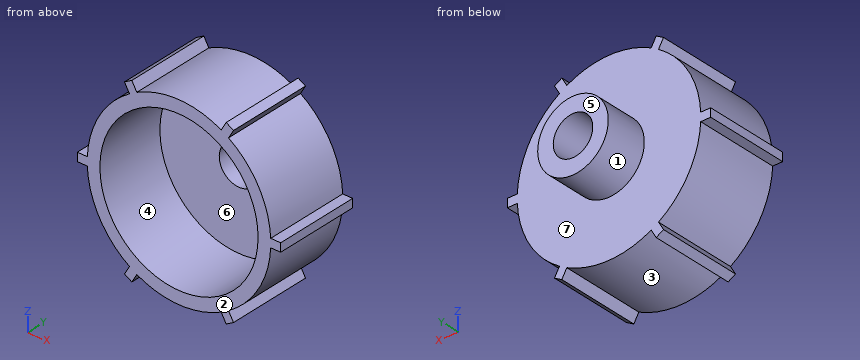
Autodesk Inventor part; units mm, degrees
ref_plane "YZ Plane" through (0, 0, 0) normal (1, 0, 0) x (0, 1, 0)
ref_plane "XZ Plane" through (0, 0, 0) normal (0, 1, 0) x (-1, 0, 0)
ref_plane "XY Plane" through (0, 0, 0) normal (0, 0, 1) x (1, 0, 0)
sketch "スケッチ1" plane through (0, 0, 0) normal (0, 1, 0) x (-1, 0, 0)
  circle A0 centre (0, 0) radius 6.5
  line L0 (0, 0) -> (0, -6.5) construction
  line L1 (3.5063, -5.4732) -> (2.9867, -5.7732)
  line L2 (2.9867, -5.7732) -> (3.3402, -6.3854)
  line L3 (3.3402, -6.3854) -> (3.8598, -6.0854)
  line L4 (3.8598, -6.0854) -> (3.5063, -5.4732)
  line L5 (0, 0) -> (3.6, -6.2354) construction
  line L6 (6.4931, 0.3) -> (6.4931, -0.3)
  line L7 (6.4931, -0.3) -> (7.2, -0.3)
  line L8 (7.2, -0.3) -> (7.2, 0.3)
  line L9 (7.2, 0.3) -> (6.4931, 0.3)
  line L10 (0, 0) -> (7.2, 0) construction
  line L11 (2.9867, 5.7732) -> (3.5063, 5.4732)
  line L12 (3.5063, 5.4732) -> (3.8598, 6.0854)
  line L13 (3.8598, 6.0854) -> (3.3402, 6.3854)
  line L14 (3.3402, 6.3854) -> (2.9867, 5.7732)
  line L15 (0, 0) -> (3.6, 6.2354) construction
  line L16 (-3.5063, 5.4732) -> (-2.9867, 5.7732)
  line L17 (-2.9867, 5.7732) -> (-3.3402, 6.3854)
  line L18 (-3.3402, 6.3854) -> (-3.8598, 6.0854)
  line L19 (-3.8598, 6.0854) -> (-3.5063, 5.4732)
  line L20 (0, 0) -> (-3.6, 6.2354) construction
  line L21 (-6.4931, -0.3) -> (-6.4931, 0.3)
  line L22 (0, 0) -> (-7.2, 0) construction
  line L23 (-6.4931, 0.3) -> (-7.2, 0.3)
  line L24 (-7.2, -0.3) -> (-6.4931, -0.3)
  line L25 (-7.2, 0.3) -> (-7.2, -0.3)
  line L26 (0, 0) -> (-3.6, -6.2354) construction
  line L27 (-2.9867, -5.7732) -> (-3.5063, -5.4732)
  line L28 (-3.5063, -5.4732) -> (-3.8598, -6.0854)
  line L29 (-3.8598, -6.0854) -> (-3.3402, -6.3854)
  line L30 (-3.3402, -6.3854) -> (-2.9867, -5.7732)
  dimension "d0" = 13
  dimension "d3" = 30
  dimension "d4" = 7.2
  dimension "d6" = 0.6
  dimension "d7" = 7.2
  dimension "d8" = 0.6
  dimension "d9" = 90
  dimension "d10" = 7.2
  dimension "d11" = 0.6
  dimension "d12" = 150
  dimension "d13" = 7.2
  dimension "d14" = 0.6
  dimension "d15" = 7.2
  dimension "d16" = 0.6
  dimension "d17" = 7.2
  dimension "d18" = 0.6
  dimension "d19" = 30
  dimension "d20" = 90
  dimension "d21" = 150
extrude "押し出し1" add sketch "スケッチ1" along normal blind 6
sketch "スケッチ2" plane through (0, 6, 0) normal (0, 1, 0) x (1, 0, 0)
  circle A0 centre (0, 0) radius 2.5
  dimension "d24" = 5
extrude "押し出し2" add sketch "スケッチ2" along normal blind 3
sketch "スケッチ3" plane through (0, 9, 0) normal (0, 1, 0) x (1, 0, 0)
  point P0 (0, 0)
  point P1 (0, 0)
hole "穴1" at (0, 9, 0) direction (0, -1, 0) diameter 2.8 end through all
sketch "スケッチ4" plane through (0, 0, 0) normal (0, -1, 0) x (1, 0, 0)
  circle A0 centre (0, 0) radius 5.6
  dimension "d34" = 11.2
extrude "押し出し3" cut sketch "スケッチ4" against normal blind 5
properties part number "CamCap_holder"
Can you work these out from the model? Positions are in its coordinate system, mm. Face numbers are marked on the shaded views. A direction names the side the tool comes from. Round coordinates to 2 decimals unless told otherwise and drop trailing zeros. Order: outer loops, then holes, each group sorted by start corner. A loop starts at its lowest first (then second) coordinate and runs counter-clockwise, first axis right, second up. Notation, with made-up numbers: M 17.25,86.25 L 28.25,86.25 A34 ccw 28.25,121.25 Z; hole C 83.25,-25.75 d5. An arc over 180 degrees is marked long. Use a Markdown table: item, result.
1) If I drill on line 1 along Z through (x, y) = (0, 7.55); line 2 along X through (y, z) = (5, -6), over which ranges is the centre line in solid material (lowest first)?
Geometry says:
| item | result |
|---|---|
| line 1 | z = -2.5 to -1.4, 1.4 to 2.5 |
| line 2 | x = -3.81 to -3.12, -2.5 to 2.5, 3.12 to 3.81 |
2) I'm going to push flat-ended pins straight in: P1, Ø3, axis at y = 8, z = -4.5, coming from the +X side; P2, Ø2, axis at y = 6.5, z = -2, coming from the -X side; P3, Ø2, axis at y = 6, z = 4, coming from the -X side; P4, Ø0.8, axis at x = 7, y = 3.5, coming from the -Z side. Where does each tip first touch, or does it pass through?
Geometry says:
| item | result |
|---|---|
| P1 | passes through |
| P2 | stops at x = -6.4 |
| P3 | stops at x = -5.77 |
| P4 | stops at z = -0.3 |
3) Imagine slicing it at B-B (z = 0). List the corners of the cut face in (x, y) for me.
Geometry says:
| item | result |
|---|---|
| outline | M -7.2,0 L -5.6,0 L -5.6,5 L -1.4,5 L -1.4,9 L -2.5,9 L -2.5,6 L -7.2,6 Z; M 1.4,5 L 5.6,5 L 5.6,0 L 7.2,0 L 7.2,6 L 2.5,6 L 2.5,9 L 1.4,9 Z |
4) If we mould it in two halves opening along Z, with no side actions, what happens to the marked faces 1, 2, 3 and 4? For each: +Z half, -Z half, draft (parallel to the pull), parting line (faces both ways), or undercut.
Geometry says:
| item | result |
|---|---|
| face 1 | parting line |
| face 2 | draft |
| face 3 | -Z half |
| face 4 | undercut |
5) On a 3-axis mill with a long thin cutter (end or side, diameter ignored), from which of +Z, -Z, +X, -X, +Y, -Y can I reach the whole of each face in a straight line? I mean the marked faces 5, 6 and 7. Say none if no direction works.
Geometry says:
| item | result |
|---|---|
| face 5 | +Z, -Z, +X, -X, +Y |
| face 6 | -Y |
| face 7 | +Y |
6) Imagine slicing it at C-C (y = 1.75). List the corners of the cut face in (x, z) for me, then the cut area to 3 significant figures.
Geometry says:
| item | result |
|---|---|
| outline | M -7.2,-0.3 L -6.49,-0.3 A6.5 ccw -3.51,-5.47 L -3.86,-6.09 L -3.34,-6.39 L -2.99,-5.77 A6.5 ccw 2.99,-5.77 L 3.34,-6.39 L 3.86,-6.09 L 3.51,-5.47 A6.5 ccw 6.49,-0.3 L 7.2,-0.3 L 7.2,0.3 L 6.49,0.3 A6.5 ccw 3.51,5.47 L 3.86,6.09 L 3.34,6.39 L 2.99,5.77 A6.5 ccw -2.99,5.77 L -3.34,6.39 L -3.86,6.09 L -3.51,5.47 A6.5 ccw -6.49,0.3 L -7.2,0.3 Z; hole C 0,0 d11.2 |
| area | 36.7 mm² |
7) Imagine slicing it at A-A (x = 0). List the corners of the cut face in (y, z) for me.
Geometry says:
| item | result |
|---|---|
| outline | M 0,-6.5 L 6,-6.5 L 6,-2.5 L 9,-2.5 L 9,-1.4 L 5,-1.4 L 5,-5.6 L 0,-5.6 Z; M 0,5.6 L 5,5.6 L 5,1.4 L 9,1.4 L 9,2.5 L 6,2.5 L 6,6.5 L 0,6.5 Z |
8) Imagine slicing it at D-D (z = -3.5). List the corners of the cut face in (x, y) for me, then the cut area to 3 significant figures.
Geometry says:
| item | result |
|---|---|
| outline | M -5.48,0 L -4.37,0 L -4.37,5 L 4.37,5 L 4.37,0 L 5.48,0 L 5.48,6 L -5.48,6 Z |
| area | 22.0 mm² |
